Can you work these out from the drawing? Everything is in mm from the part's minimum corner. A direction names the side the tool comes from. Coordinates: 2 decimals unless noted, no trailing zeros. Loops run counter-clockwise (first coordinate to the right, second up) from the corner with the lowest first, then second, coordinate; pieces in that order, holes last.
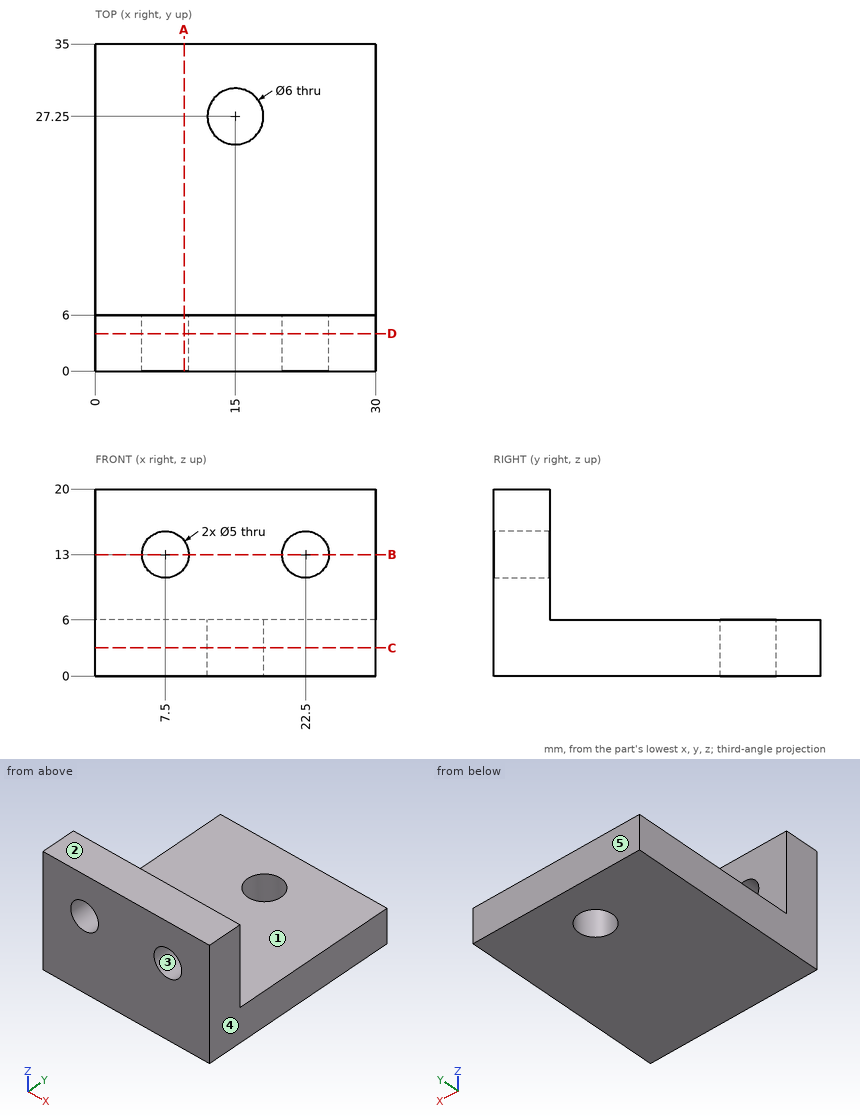
Item 1: On a 3-axis mill with a long thin cutter (end or side, diameter ignored), from which of +Z, -Z, +X, -X, +Y, -Y can I reach the whole of each face in a straight line? I mean the marked faces 1 and 2. Say none if no direction works.
Results are:
face 1: +Z, +X, -X, +Y
face 2: +Z, +X, -X, +Y, -Y
Item 2: Suppose I cut it at A-A, the plane x = 9.5. Please give me the cut outline in (y, z), plus the area to 3 significant figures.
Results are:
outline: (0, 0) - (35, 0) - (35, 6) - (6, 6) - (6, 11.5) - (0, 11.5) - close; (0, 14.5) - (6, 14.5) - (6, 20) - (0, 20) - close
area: 276 mm2
Item 3: We'd pull the mould along X, two halves only. Please class the marked faces 3, 4 and 5: +X half, -X half, draft (parallel to the pull), parting line (faces both ways), or undercut.
Results are:
face 3: undercut
face 4: +X half
face 5: draft
Item 4: Suppose I cut it at B-B, the plane z = 13. Please give me the cut outline in (x, y), plus the area to 3 significant figures.
Results are:
outline: (0, 0) - (5, 0) - (5, 6) - (0, 6) - close; (10, 0) - (20, 0) - (20, 6) - (10, 6) - close; (25, 0) - (30, 0) - (30, 6) - (25, 6) - close
area: 120 mm2
Item 5: I'm going to push flat-ended pins straight in: P1, Ø7, axis at x = 13.5, z = 14, coming from the +Y side; P2, Ø14.5, axis at x = 22, y = 19.5, coming from the +Z side. Where does each tip first touch, or does it pass through?
Results are:
P1: stops at y = 6
P2: stops at z = 6
Item 6: Suppose I cut it at C-C, the plane z = 3. Please give me the cut outline in (x, y).
Results are:
outline: (0, 0) - (30, 0) - (30, 35) - (0, 35) - close; hole circle Ø6 at (15, 27.25)
Item 7: Suppose I cut it at D-D, the plane y = 4. Please give me the cut outline in (x, z), plus the area to 3 significant figures.
Results are:
outline: (0, 0) - (30, 0) - (30, 20) - (0, 20) - close; hole circle Ø5 at (7.5, 13); hole circle Ø5 at (22.5, 13)
area: 561 mm2
Item 8: I need wall thicknesses on line 1 along X through (y, z) = (3.2, 13); line 2 along Y through (x, z) = (15, 4.6); line 3 along Z through (x, y) = (2.75, 9). Which ranges of each line are inside material? Lowest first, please.
Results are:
line 1: x = 0 to 5, 10 to 20, 25 to 30
line 2: y = 0 to 24.25, 30.25 to 35
line 3: z = 0 to 6
